Answer from the drawing. Dimensions are ordinates in mm from the lowest x, y and z of the part. A direction names the side the tool comes from. Give positions to 0.01 mm unless a question says otherwise; leave off trailing zeros. Order: outer loops, then holes, each group sorted by start corner. A loop starts at its lowest first (then second) coordinate and runs counter-clockwise, first axis right, second up. Notation, with made-up numbers: M 32.25,40 L 56.25,40 A23 ccw 56.25,59 Z; hole C 63,8 d9. An arc over 180 degrees is marked long. One line per item, written item: value.
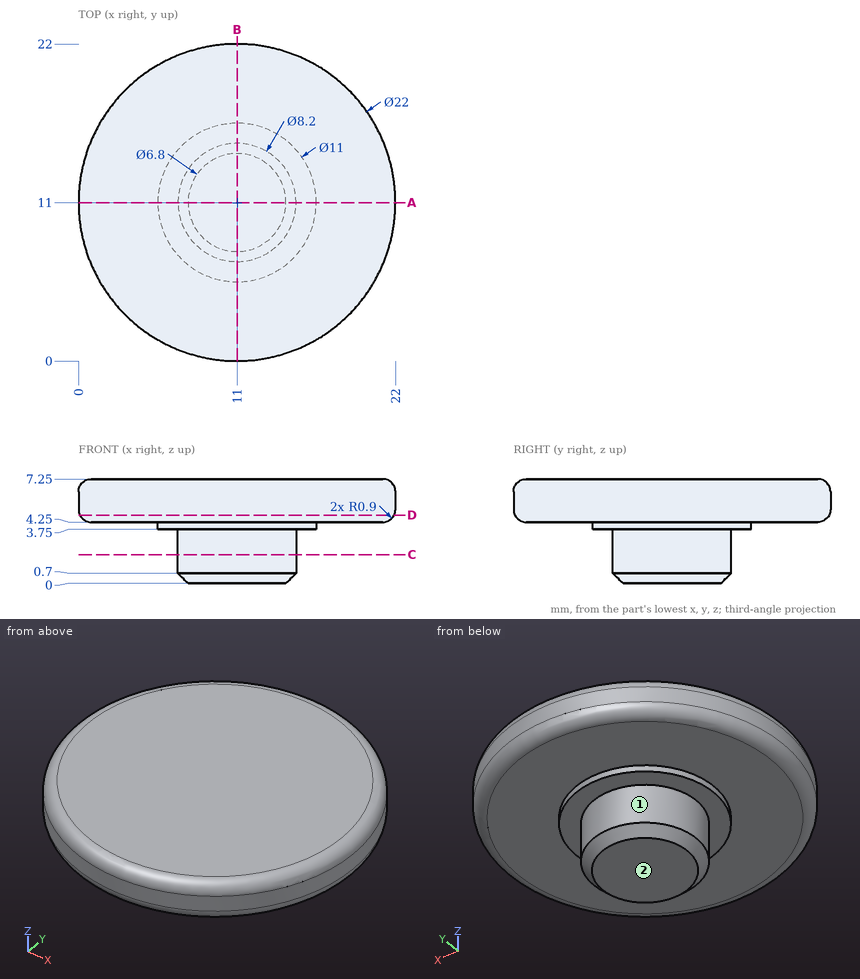
(1) Given P1, Ø4, axis at y = 18, z = 3.5, coming from the +X side; P2, Ø2, axis at x = 2.5, z = 6.5, coming from the -Y side, each flat-ended and moving along its own axis, determine where each tip first touches the part or whether it passes through.
Findings:
P1: stops at x = 20.46
P2: stops at y = 2.96
(2) Section A-A, the plane y = 11 is taken. Give the vertices of the cut face in (x, z).
Findings:
outline: M 0,5.15 A0.9 ccw 0.9,4.25 L 5.5,4.25 L 5.5,3.75 L 6.9,3.75 L 6.9,0.7 L 7.6,0 L 14.4,0 L 15.1,0.7 L 15.1,3.75 L 16.5,3.75 L 16.5,4.25 L 21.1,4.25 A0.9 ccw 22,5.15 L 22,6.35 A0.9 ccw 21.1,7.25 L 0.9,7.25 A0.9 ccw 0,6.35 Z
(3) Section C-C, the plane z = 2 is taken. Give the vertices of the cut face in (x, y), then the cut area to 3 significant figures.
Findings:
outline: C 11,11 d8.2
area: 52.8 mm^2
(4) Section D-D, the plane z = 4.75 is taken. Give the vertices of the cut face in (x, y).
Findings:
outline: C 11,11 d21.81
(5) Find the intervals of material crossed by probe 1 along Z at (x, y) = (15, 18); probe 2 along Y at (x, z) = (10.25, 1.25); probe 3 along X at (y, z) = (11.5, 3.5), in increasing order. Write a range as from..to.
Findings:
probe 1: z = 4.25..7.25
probe 2: y = 6.97..15.03
probe 3: x = 6.93..15.07
(6) Which of the six approach directions +Z, -Z, +X, -X, +Y, -Y give full straight-line access (tool end or side, diameter ignored) to the marked faces 1 and 2?
Findings:
face 1: -Z
face 2: -Z, +X, -X, +Y, -Y
